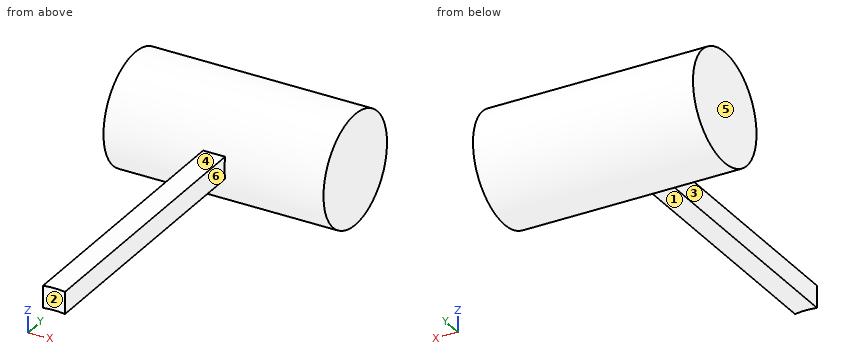
from build123d import *

# Parameters (mm, degrees)
SKETCH1_R           = 5
BOSS_EXTRUDE1_DEPTH = 10
BOSS_EXTRUDE2_DEPTH = 1


with BuildPart() as part:
    # Sketch1 → Boss-Extrude1 (new, symmetric)
    with BuildSketch(Plane(origin=(0, 0, 0), x_dir=(0, 0, -1), z_dir=(1, 0, 0))):
        Circle(SKETCH1_R)
    extrude(amount=BOSS_EXTRUDE1_DEPTH, both=True)

    # Sketch2 → Boss-Extrude2 (add, symmetric)
    with BuildSketch(Plane.XY):
        with BuildLine():
            Line((1, 0), (-1, 0))
            Line((-1, 0), (-1, -30.101020514))
            ThreePointArc((-1, -30.101020514), (0, -30), (1, -30.101020514))
            Line((1, -30.101020514), (1, 0))
        make_face()
    extrude(amount=BOSS_EXTRUDE2_DEPTH, both=True)


solid = part.part
Input: part model. Units: mm. Frame: model coordinates. Face numbers are marked on the shaded views. A direction names the side the tool comes from. Give positions to 0.01 mm unless a question says otherwise; leave off trailing zeros. Loops run counter-clockwise (first coordinate to the right, second up) from the corner with the lowest first, then second, coordinate; pieces in that order, holes last. Notation, with made-up numbers: (-33.75, 67.25) - (-17.75, 67.25) arc R28 cw to (-17.75, 87.25) - close; hole circle Ø9 at (23, 58). An arc over 180 degrees is marked (long way). Use CSV: the item, a comma, the result in double quotes. Start each with the question number.
Item 1: Section C-C on y = -10. Return loops of the section in (x, z), then the cut area to 3 significant figures.
Item 2: Mould query, pull axis X, two halves, no side actions, for the marked faces 1, 2 and 3. Classes: pulls with the +X half, pulls with the -X half, needs draft (parallel to the pull), parting line crosses it, or undercut.
Item 3: Reachability of the marked faces 4, 5 and 6 from +Z, -Z, +X, -X, +Y, -Y: full face, straight path, thin tool, end or side. Return the list, or none.
Item 4: Line query: line 1 (Z direction, x = 0.75, y = -18.5); line 2 (Z direction, x = 4.5, y = -2). Output: solid intervals per line, ascending.
Item 5: Section A-A on z = 0. Return loops of the section in (x, y).
Item 6: Section B-B on x = -2.75. Return loops of the section in (y, z).
Item 7: Contact query for flat-ended pins moving along their axis: P1, Ø2, axis at x = -5, y = -6.5, coming from the +Z side; P2, Ø1.6, axis at y = -20.5, z = 0, coming from the -X side; P3, Ø1.6, axis at x = 0, y = -17, coming from the +Z side; P4, Ø1.5, axis at x = -0.5, z = -3, coming from the +Y side. Output: stop coordinate, or through.
Item 8: Section D-D on x = 0. Return loops of the section in (y, z).
Ans:
1,outline,"(-1, -1) - (1, -1) - (1, 1) - (-1, 1) - close"
1,area,"4.00 mm2"
2,face 1,"needs draft"
2,face 2,"undercut"
2,face 3,"pulls with the -X half"
3,face 4,"+Z, +X, -X, -Y"
3,face 5,"+Z, -Z, -X, +Y, -Y"
3,face 6,"+Z, -Z, +X, -Y"
4,line 1,"z = -1 to 1"
4,line 2,"z = -4.58 to 4.58"
5,outline,"(-10, -5) - (-1, -5) - (-1, -30.1) arc R5 cw to (1, -30.1) - (1, -5) - (10, -5) - (10, 5) - (-10, 5) - close"
6,outline,"circle Ø10 at (0, 0)"
7,P1,"passes through"
7,P2,"stops at x = -1"
7,P3,"stops at z = 1"
7,P4,"stops at y = 4.47"
8,outline,"(-30, -1) - (-4.9, -1) arc R5 ccw (long way) to (-4.9, 1) - (-30, 1) - close"
